from build123d import *

# Parameters (mm, degrees)
SKETCH1_R                                       = 12.446
SKETCH1_R_2                                     = 1.27
BOSS_EXTRUDE1_DEPTH                             = 24.892
CSK_FOR_M3_FLAT_HEAD_MACHINE_SCREW1_D           = 3.4
CSK_FOR_M3_FLAT_HEAD_MACHINE_SCREW1_CSINK_D     = 6.3
CSK_FOR_M3_FLAT_HEAD_MACHINE_SCREW1_CSINK_ANGLE = 90
SKETCH5_R                                       = 12.192
BOSS_EXTRUDE2_DEPTH                             = 30.734
SKETCH6_R                                       = 3.556
BOSS_EXTRUDE3_DEPTH                             = 2.54
SKETCH7_R                                       = 2.032
BOSS_EXTRUDE4_DEPTH                             = 9.906
SKETCH8_W                                       = 2.032
SKETCH8_H                                       = 0.254
CUT_EXTRUDE2_DEPTH                              = 9.906
SKETCH9_R                                       = 3.175
BOSS_EXTRUDE5_DEPTH                             = 1.524
SKETCH10_W                                      = 2.032
SKETCH10_H                                      = 0.254
BOSS_EXTRUDE6_DEPTH                             = 4.318


with BuildPart() as part:
    # Sketch1 → Boss-Extrude1 (new body)
    with BuildSketch(Plane(origin=(0, 0, 0), x_dir=(1, 0, 0), z_dir=(0, 1, 0))):
        Circle(SKETCH1_R)
        with Locations((-9.017, 0)):
            Circle(SKETCH1_R_2, mode=Mode.SUBTRACT)
        with Locations((9.017, 0)):
            Circle(SKETCH1_R_2, mode=Mode.SUBTRACT)
    extrude(amount=BOSS_EXTRUDE1_DEPTH)

    # CSK for M3 Flat Head Machine Screw1 (through all)
    with Locations(Plane(origin=(0, 24.892, 0), x_dir=(1, 0, 0), z_dir=(0, 1, 0))):
        with Locations((0, 8.119865968), (0, -7.587036194)):
            CounterSinkHole(CSK_FOR_M3_FLAT_HEAD_MACHINE_SCREW1_D / 2, CSK_FOR_M3_FLAT_HEAD_MACHINE_SCREW1_CSINK_D / 2, counter_sink_angle=CSK_FOR_M3_FLAT_HEAD_MACHINE_SCREW1_CSINK_ANGLE)

    # Sketch5 → Boss-Extrude2 (add)
    with BuildSketch(Plane(origin=(0, 24.892, 0), x_dir=(1, 0, 0), z_dir=(0, 1, 0))):
        Circle(SKETCH5_R)
    extrude(amount=BOSS_EXTRUDE2_DEPTH)

    # Sketch6 → Boss-Extrude3 (add)
    with BuildSketch(Plane(origin=(0, 0, 0), x_dir=(1, 0, 0), z_dir=(0, 1, 0))):
        Circle(SKETCH6_R)
    extrude(amount=-BOSS_EXTRUDE3_DEPTH)

    # Sketch7 → Boss-Extrude4 (add)
    with BuildSketch(Plane(origin=(0, -2.54, 0), x_dir=(-1, 0, 0), z_dir=(0, -1, 0))):
        Circle(SKETCH7_R)
    extrude(amount=BOSS_EXTRUDE4_DEPTH)

    # Sketch8 → Cut-Extrude2 (cut)
    with BuildSketch(Plane(origin=(0, -12.446, 0), x_dir=(-1, 0, 0), z_dir=(0, -1, 0))):
        with Locations((0, -1.905)):
            Rectangle(SKETCH8_W, SKETCH8_H)
        with Locations((0, 1.905)):
            Rectangle(SKETCH8_W, SKETCH8_H)
    extrude(amount=-CUT_EXTRUDE2_DEPTH, mode=Mode.SUBTRACT)

    # Sketch9 → Boss-Extrude5 (add)
    with BuildSketch(Plane(origin=(0, 55.626, 0), x_dir=(1, 0, 0), z_dir=(0, 1, 0))):
        Circle(SKETCH9_R)
    extrude(amount=BOSS_EXTRUDE5_DEPTH)

    # Sketch10 → Boss-Extrude6 (add)
    with BuildSketch(Plane(origin=(0, 55.626, 0), x_dir=(1, 0, 0), z_dir=(0, 1, 0))):
        with Locations((-9.017, 0)):
            Rectangle(SKETCH10_W, SKETCH10_H)
        with Locations((9.017, 0)):
            Rectangle(SKETCH10_W, SKETCH10_H)
    extrude(amount=BOSS_EXTRUDE6_DEPTH)


solid = part.part
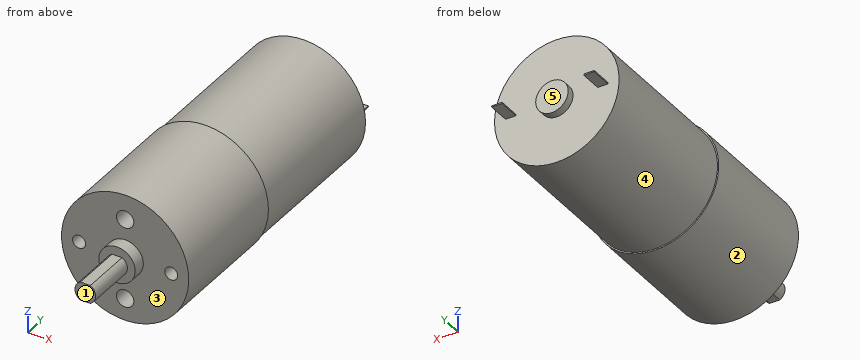
Part model, mm, in its own coordinate system. Face numbers are marked on the shaded views. A direction names the side the tool comes from. Coordinates: 2 decimals unless noted, no trailing zeros. Order: outer loops, then holes, each group sorted by start corner. A loop starts at its lowest first (then second) coordinate and runs counter-clockwise, first axis right, second up. Notation, with made-up numbers: (78, 51.25) - (115, 51.25) arc R7 ccw to (115, 55.25) - close; hole circle Ø10 at (-11, 31). An arc over 180 degrees is marked (long way). Use CSV: the item, a comma, the result in double quotes.
Item 1: Saw through at B-B on z = -2.5. Give the cut face in (x, y).
Solved:
outline,"(-12.19, 0) - (-2.53, 0) - (-2.53, -2.54) - (2.53, -2.54) - (2.53, 0) - (12.19, 0) - (12.19, 24.89) - (11.93, 24.89) - (11.93, 55.63) - (1.96, 55.63) - (1.96, 57.15) - (-1.96, 57.15) - (-1.96, 55.63) - (-11.93, 55.63) - (-11.93, 24.89) - (-12.19, 24.89) - close"
Item 2: Saw through at D-D on y = 45.5. Give the cut face in (x, z).
Solved:
outline,"circle Ø24.38 at (0, 0)"
Item 3: Probe probe 1 along X at (y, z) = (18.5, 0); probe 2 along Z at (x, y) = (0, 13.75); probe 3 along Y at (x, z) = (0.25, 6.5). List the from-to ranges inside material, lowest first.
Solved:
probe 1,"x = -12.45 to -10.29, -7.75 to 7.75, 10.29 to 12.45"
probe 2,"z = -12.45 to -9.82, -6.42 to 5.89, 9.29 to 12.45"
probe 3,"y = 24.89 to 55.63"
Item 4: Saw through at C-C on y = 22.5. Give the cut face in (x, z), and give its area (3 significant figures).
Solved:
outline,"circle Ø24.89 at (0, 0); hole circle Ø2.54 at (-9.02, 0); hole circle Ø3.4 at (0, -8.12); hole circle Ø3.4 at (0, 7.59); hole circle Ø2.54 at (9.02, 0)"
area,"458 mm²"
Item 5: Drop flat-ended pins along their axis: P1, Ø4, axis at y = 13.5, z = 2, coming from the -X side; P2, Ø10, axis at x = 1, y = 41.5, coming from the -Z side; P3, Ø5, axis at x = 0.5, z = 8, coming from the -Y side; P4, Ø7.5, axis at x = -0.5, z = -1, coming from the +Y side. Give the stop position or say it passes through.
Solved:
P1,"stops at x = -12.45"
P2,"stops at z = -12.19"
P3,"stops at y = 0"
P4,"stops at y = 57.15"
Item 6: 3-axis set-ups, long thin cutter, end or side, ignore diameter. For the marked faces 1, 2, 3, 4 and 5: which of +Z, -Z, +X, -X, +Y, -Y reach the whole face in a straight line?
Solved:
face 1,"+Z, -Z, +X, -X, -Y"
face 2,"+Y, -Y"
face 3,"-Y"
face 4,"+Y"
face 5,"+Z, -Z, +Y"
